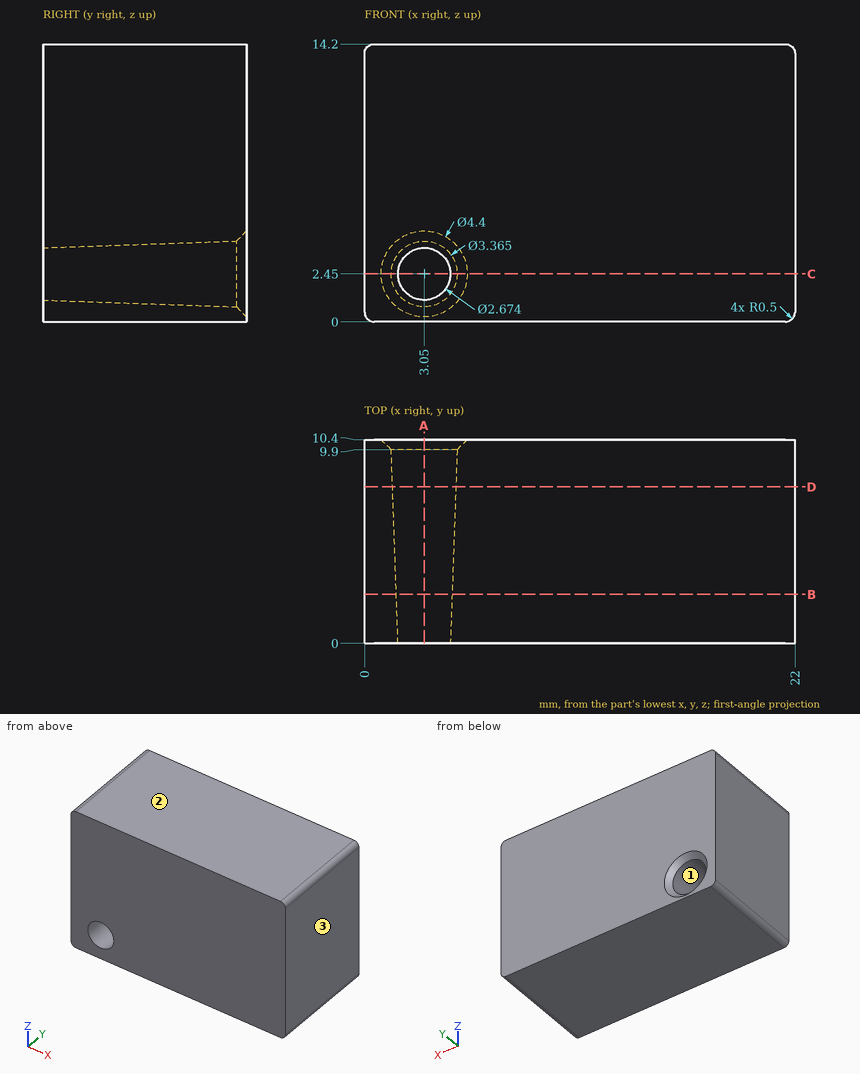
Could you check a few things on this drawing? It's one solid part, dimensions in mm from its lowest x, y, z. Coordinates: 2 decimals unless noted, no trailing zeros. Loops run counter-clockwise (first coordinate to the right, second up) from the corner with the lowest first, then second, coordinate; pieces in that order, holes last.
1. Imagine slicing it at D-D (y = 8). Please give me the cut outline in (x, z).
2. Imagine slicing it at B-B (y = 2.5). Please give me the cut outline in (x, z).
3. Imagine slicing it at C-C (z = 2.45). Please give me the cut outline in (x, y), and give its area (3 significant figures).
4. Imagine slicing it at A-A (x = 3.05). Please give me the cut outline in (y, z), and give its area (3 significant figures).
5. We'd pull the mould along X, two halves only. Please class the marked faces 1, 2 and 3: released by +X, released by -X, zero draft, split by the parting line, or undercut.
6. I need wall thicknesses on L1, parallel to Z at x = 3, y = 9.75; L2, parallel to X at y = 6.75, z = 3; L3, parallel to Z at x = 4, y = 1.5 (1 decimal). Which ranges of each line are inside material? Lowest first, please.
7. For P1, Ø1.5, axis at y = 1.5, z = 5.5, coming from the -X side, with a flat end and sliding along its axis, tell me the tip position at first contact or that it passes through.
Computed values:
1. outline: (0, 0.5) arc R0.5 ccw to (0.5, 0) - (21.5, 0) arc R0.5 ccw to (22, 0.5) - (22, 13.7) arc R0.5 ccw to (21.5, 14.2) - (0.5, 14.2) arc R0.5 ccw to (0, 13.7) - close; hole circle Ø3.23 at (3.05, 2.45)
2. outline: (0, 0.5) arc R0.5 ccw to (0.5, 0) - (21.5, 0) arc R0.5 ccw to (22, 0.5) - (22, 13.7) arc R0.5 ccw to (21.5, 14.2) - (0.5, 14.2) arc R0.5 ccw to (0, 13.7) - close; hole circle Ø2.85 at (3.05, 2.45)
3. outline: (0, 0) - (1.71, 0) - (1.37, 9.9) - (0.85, 10.4) - (0, 10.4) - close; (4.39, 0) - (22, 0) - (22, 10.4) - (5.25, 10.4) - (4.73, 9.9) - close
3. area: 197 mm2
4. outline: (0, 0) - (10.4, 0) - (10.4, 0.25) - (9.9, 0.77) - (0, 1.11) - close; (0, 3.79) - (9.9, 4.13) - (10.4, 4.65) - (10.4, 14.2) - (0, 14.2) - close
4. area: 116 mm2
5. face 1: undercut
5. face 2: zero draft
5. face 3: released by +X
6. L1: z = 0 to 0.77, 4.13 to 14.2
6. L2: x = 0 to 1.58, 4.52 to 22
6. L3: z = 0 to 1.4, 3.5 to 14.2
7. P1: stops at x = 0
